Check sheet for the drawn part. Datum: minimum x, y, z corner. Units: mm. A direction names the side the tool comes from. Round coordinates to 2 decimals unless told otherwise and drop trailing zeros. Order: outer loops, then holes, each group sorted by start corner. A loop starts at its lowest first (then second) coordinate and runs counter-clockwise, first axis right, second up.
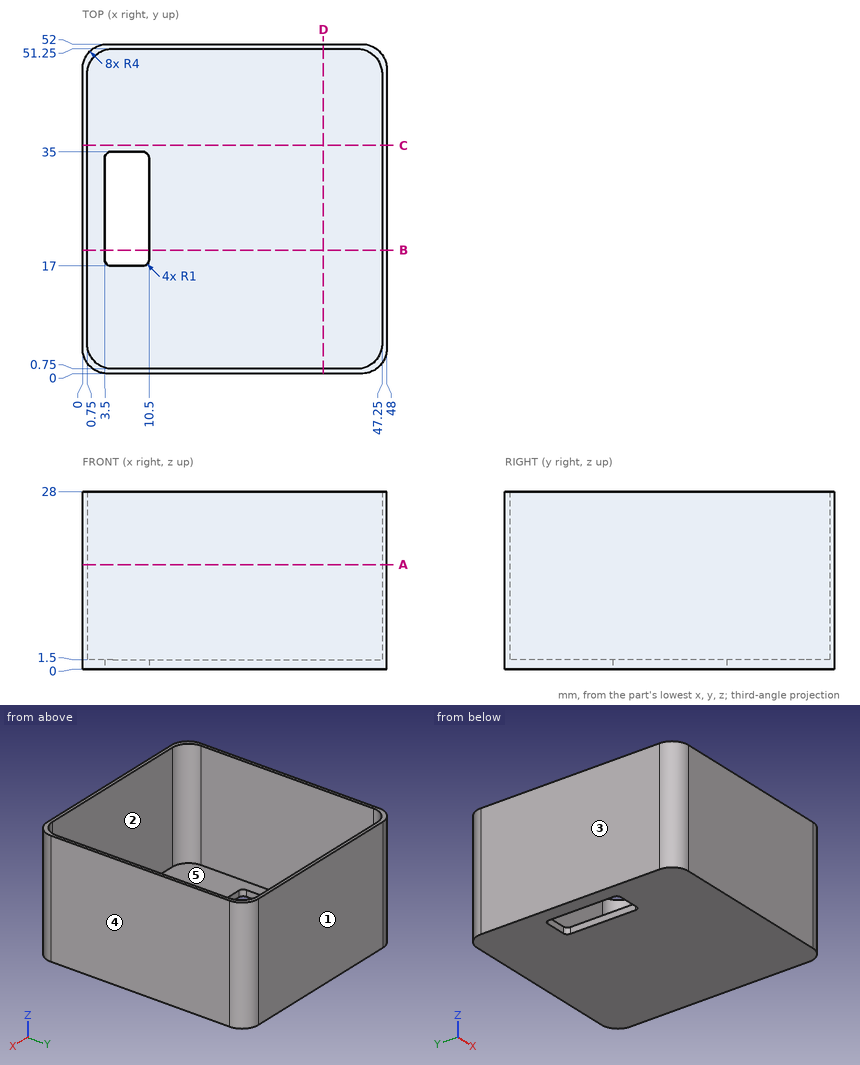
(1) Draft check along Y on the marked faces 1, 2 and 3. Enter one of: released by +Y, released by -Y, zero draft, split by the parting line, or undercut.
Returned:
face 1: released by +Y
face 2: undercut
face 3: zero draft
(2) Depth check by flat-ended pin: P1, Ø2, axis at x = 35.5, y = 13.5, coming from the -Z side; P2, Ø1.5, axis at x = 36.5, y = 46, coming from the +Z side. Enter the tip coordinate at first touch or a pass-through.
Returned:
P1: stops at z = 0
P2: stops at z = 1.5
(3) Sectioned sample at B-B, the plane y = 19.5. Record the cut outline in (x, z).
Returned:
outline: (0, 0) - (3.5, 0) - (3.5, 1.5) - (0.75, 1.5) - (0.75, 28) - (0, 28) - close; (10.5, 0) - (48, 0) - (48, 28) - (47.25, 28) - (47.25, 1.5) - (10.5, 1.5) - close
(4) Sectioned sample at A-A, the plane z = 16.5. Record the cut outline in (x, y), and give its area (3 significant figures).
Returned:
outline: (0, 4) arc R4 ccw to (4, 0) - (44, 0) arc R4 ccw to (48, 4) - (48, 48) arc R4 ccw to (44, 52) - (4, 52) arc R4 ccw to (0, 48) - close; hole (0.75, 4.75) arc R4 ccw to (4.75, 0.75) - (43.25, 0.75) arc R4 ccw to (47.25, 4.75) - (47.25, 47.25) arc R4 ccw to (43.25, 51.25) - (4.75, 51.25) arc R4 ccw to (0.75, 47.25) - close
area: 148 mm2
(5) Material ranges on line 1 (X direction, y = 10, z = 12); line 2 (Y direction, x = 16, z = 22.25); line 3 (Z direction, x = 35.5, y = 49.5), recorded low to high.
Returned:
line 1: x = 0 to 0.75, 47.25 to 48
line 2: y = 0 to 0.75, 51.25 to 52
line 3: z = 0 to 1.5
(6) Sectioned sample at C-C, the plane y = 36. Record the cut outline in (x, z), and give its area (3 significant figures).
Returned:
outline: (0, 0) - (48, 0) - (48, 28) - (47.25, 28) - (47.25, 1.5) - (0.75, 1.5) - (0.75, 28) - (0, 28) - close
area: 112 mm2
(7) Sectioned sample at D-D, the plane x = 38. Record the cut outline in (y, z), and give its area (3 significant figures).
Returned:
outline: (0, 0) - (52, 0) - (52, 28) - (51.25, 28) - (51.25, 1.5) - (0.75, 1.5) - (0.75, 28) - (0, 28) - close
area: 118 mm2
(8) Set-up check for the marked faces 4 and 5: record each of +Z, -Z, +X, -X, +Y, -Y from which the full face is reachable in a straight line by a thin tool's end or side.
Returned:
face 4: +Z, -Z, +X, +Y, -Y
face 5: +Z
